Geometry: final body of the model. Coordinates: model frame, mm. A direction names the side the tool comes from. Give positions to 0.01 mm unless a question says otherwise; leave off trailing zeros. Write each loop counter-clockwise with the first axis right and the second up, starting at its lowest first coordinate (ties: lowest second). Pieces come first, ordered by that corner, then holes. Notation, with made-up numbers: (35, -14.75) -> (61, -14.75) arc R24 cw to (61, 2.25) -> close; hole circle Ø4 at (-13.5, 41.25). An arc over 180 degrees is marked (long way). Answer in a Markdown table with one row per item. Add a question column.
Item 1: Draft query along Z for faces 5 (the flat face through (-19, -3, 2.108)), 6 (the flat face through (1, -11, 1.524)), 7 (the cylindrical face through (-18.936, -0.093, 7.645)), 8 (the flat face through (-23.05, -4, 1)). Return one class per face: +Z half, -Z half, draft (parallel to the pull), parting line (faces both ways), or undercut.
Item 2: Section query A-A on z = 6.75. Output: boundary loops of the cut face in (x, y).
Item 3: First-contact query: P1, Ø1.8, axis at x = 0, y = -3.76, coming from the +Z side; P2, Ø2, axis at y = -2, z = 4, coming from the -X side; P3, Ø1.1, axis at x = -0.5, y = -10.5, coming from the -Z side; P4, Ø2, axis at x = -16, z = 3.5, coming from the -Y side. Flat tips, straight axial feed; report the tip coordinate or a pass-through.
Item 4: Material intervals for probe 1 along Y at (x, z) = (0, 0.5); probe 2 along Z at (x, y) = (-12.5, -1.75); probe 3 along X at (y, z) = (-0.25, 7.25), sorted ascending. Write a range as from..to.
Item 5: Section query D-D on x = 17. Output: boundary loops of the cut face in (y, z).
Item 6: Access query for faces 1 (the flat face through (-16.599, 0, 3)), 2 (the flat face through (-21.679, 0, 3)), 3 (the cylindrical face through (-19.195, -6.514, 1.812)), 4 (the cylindrical face through (-0.039, -2.007, 1.812)). Directions: +Z, -Z, +X, -X, +Y, -Y. A direction counts if a zero-diameter tool reaches every point of the face in a straight line with its end or side. Return the directions, or none.
Item 7: Section query C-C on z = 3.5. Output: boundary loops of the cut face in (x, y), plus the area to 3 significant figures.
Item 8: Section query B-B on x = 0. Output: boundary loops of the cut face in (y, z).
```python
from build123d import *

# Parameters (mm, degrees)
SKETCH_1_W          = 46.101
SKETCH_1_H          = 7.9502
EXTRUDE_1_DEPTH     = 1.524
EXTRUDE_2_DEPTH     = 0.5842
SKETCH_3_R          = 1.5621
EXTRUDE_3_DEPTH     = 0.5842
FILLET_1_R          = 0.508
SKETCH_4_R          = 0.762
CUT_EXTRUDE_4_DEPTH = 26.241699688
EXTRUDE_5_DEPTH     = 0.5842
SKETCH_6_R          = 0.762
CUT_EXTRUDE_6_DEPTH = 28.442983889


with BuildPart() as part:
    # 草圖1 → 伸長1 (new body)
    with BuildSketch(Plane.XY):
        with Locations((0, -3.9751)):
            Rectangle(SKETCH_1_W, SKETCH_1_H)
    extrude(amount=EXTRUDE_1_DEPTH)

    # 草圖2 → 伸長2 (add)
    with BuildSketch(Plane.XY.offset(1.524)):
        with BuildLine():
            Line((-21.6789, -0.381), (-21.6789, -3.9751))
            ThreePointArc((-21.6789, -3.9751), (-19.1389, -6.5151), (-16.5989, -3.9751))
            Line((-16.5989, -3.9751), (-16.5989, -0.381))
            Line((-16.5989, -0.381), (-21.6789, -0.381))
        make_face()
    extrude(amount=EXTRUDE_2_DEPTH)

    # 草圖3 → 伸長3 (add)
    with BuildSketch(Plane(origin=(0, -0.381, 0), x_dir=(1, 0, 0), z_dir=(0, 1, 0))):
        with BuildLine():
            Line((-16.5989, -1.524), (-21.6789, -1.524))
            Line((-21.6789, -1.524), (-21.6789, -6.096))
            ThreePointArc((-21.6789, -6.096), (-19.1389, -8.636), (-16.5989, -6.096))
            Line((-16.5989, -6.096), (-16.5989, -1.524))
        make_face()
        with Locations(Location((-19.1389, -6.096, 0), (0, 0, 180))):
            Circle(SKETCH_3_R, mode=Mode.SUBTRACT)
    extrude(amount=EXTRUDE_3_DEPTH)

    # 圓角1
    # the kernel refuses this fillet: 0.508 mm, written as the material it adds along each edge
    with BuildSketch(Plane(origin=(-16.5989, -0.381, 2.1082), x_dir=(0, 0, 1), z_dir=(-1, 0, 0))) as fillet_1_piece_1:
        with BuildLine():
            CenterArc((FILLET_1_R, -FILLET_1_R), FILLET_1_R, 90, 90)
            Line((0, -FILLET_1_R), (0, 0))
            Line((0, 0), (FILLET_1_R, 0))
        make_face()
    extrude(amount=5.08)
    # the kernel refuses this fillet: 0.508 mm, written as the material it takes off along each edge
    with BuildSketch(Plane(origin=(-15.5829, 0.2032, 1.524), x_dir=(0, -1.0, 2.6096797513364413e-11), z_dir=(-1, 0, 0))) as fillet_1_2_piece_1:
        with BuildLine():
            CenterArc((0.508, 0.4064), FILLET_1_R, 179.999999999, 53.130102355)
            Line((0, 0.4064), (0, 0))
            Line((0, 0), (0.2032, 0))
        make_face()
    extrude(amount=7.112, mode=Mode.SUBTRACT)

    # 草圖4 → 伸長4 (cut, through all)
    with BuildSketch(Plane.XY.offset(2.1082)):
        with Locations((-19.1389, -3.9751)):
            Circle(SKETCH_4_R)
    extrude(amount=-CUT_EXTRUDE_4_DEPTH, mode=Mode.SUBTRACT)

    # 草圖5 → 伸長5 (add)
    with BuildSketch(Plane.XY.offset(1.524)):
        with BuildLine():
            Line((-1.7526, -11.6332), (-1.7526, -3.7592))
            ThreePointArc((-1.7526, -3.7592), (0, -2.0066), (1.7526, -3.7592))
            Line((1.7526, -3.7592), (1.7526, -11.6332))
            ThreePointArc((1.7526, -11.6332), (0, -13.3858), (-1.7526, -11.6332))
        make_face()
        with BuildLine():
            Line((-0.762, -7.9502), (-0.762, -11.6332))
            ThreePointArc((-0.762, -11.6332), (0, -12.3952), (0.762, -11.6332))
            Line((0.762, -11.6332), (0.762, -7.9502))
            Line((0.762, -7.9502), (-0.762, -7.9502))
        make_face(mode=Mode.SUBTRACT)
    extrude(amount=EXTRUDE_5_DEPTH)

    # 草圖6 → 伸長6 (cut, through all)
    with BuildSketch(Plane.XY.offset(2.1082)):
        with Locations((0, -3.7592)):
            Circle(SKETCH_6_R)
    extrude(amount=-CUT_EXTRUDE_6_DEPTH, mode=Mode.SUBTRACT)


solid = part.part
```
Findings below:
| question | item | result |
|---|---|---|
| 1 | face 5 | +Z half |
| 1 | face 6 | -Z half |
| 1 | face 7 | undercut |
| 1 | face 8 | draft |
| 2 | outline | (-21.59, -0.38) -> (-20.56, -0.38) -> (-20.56, 0.2) -> (-21.59, 0.2) -> close; (-17.72, -0.38) -> (-16.68, -0.38) -> (-16.68, 0.2) -> (-17.72, 0.2) -> close |
| 3 | P1 | stops at z = 2.11 |
| 3 | P2 | passes through |
| 3 | P3 | stops at z = 1.52 |
| 3 | P4 | stops at y = -0.38 |
| 4 | probe 1 | y = -7.95..-4.52, -3..0 |
| 4 | probe 2 | z = 0..1.52 |
| 4 | probe 3 | x = -21.4..-20.19, -18.09..-16.88 |
| 5 | outline | (-7.95, 0) -> (0, 0) -> (0, 1.52) -> (-7.95, 1.52) -> close |
| 6 | face 1 | +Z, +Y, -Y |
| 6 | face 2 | +Z, -X, +Y, -Y |
| 6 | face 3 | +Z, -Y |
| 6 | face 4 | +Z, +Y |
| 7 | outline | (-21.68, -0.38) -> (-16.6, -0.38) -> (-16.6, 0.2) -> (-21.68, 0.2) -> close |
| 7 | area | 2.97 mm^2 |
| 8 | outline | (-13.39, 1.52) -> (-12.4, 1.52) -> (-12.4, 2.11) -> (-13.39, 2.11) -> close; (-7.95, 0) -> (-4.52, 0) -> (-4.52, 2.11) -> (-7.95, 2.11) -> close; (-3, 0) -> (0, 0) -> (0, 1.52) -> (-2.01, 1.52) -> (-2.01, 2.11) -> (-3, 2.11) -> close |
